Answer from the drawing. Dimensions are ordinates in mm from the lowest x, y and z of the part. Give positions to 0.01 mm unless a question says otherwise; leave off trailing zeros. Order: outer loops, then holes, each group sorted by start corner. A loop starts at its lowest first (then second) coordinate and runs counter-clockwise, first axis right, second up. Notation, with made-up numbers: (12.5, -6.5) - (22.5, -6.5) arc R17 ccw to (22.5, 23.5) - close; hole circle Ø2 at (-38, 72). An arc over 180 degrees is marked (long way). Use a Markdown table: item, result. Add a question column.
1) Find section D-D, the plane x = 190. Determine the outline of the cut face in (y, z), plus the area to 3 significant figures.
2) Find section C-C, the plane x = 99. Determine the outline of the cut face in (y, z).
3) Find section A-A, the plane y = 153. Determine the outline of the cut face in (x, z), plus the area to 3 significant figures.
4) Straight lines are drawn through the part: line 1 (X direction, y = 30.5, z = 18.25) (1 decimal); line 2 (Y direction, x = 70.5, z = 16) (1 decimal); line 3 (Y direction, x = 91, z = 14.75) (1 decimal). For each, find the intervals that lie inside material, in ascending order.
5) Flat-ended cylindrical pins translate along their axes: pin 1 (3 mm diameter, centred on x = 240, y = 183.5, fed in from +Z); pin 2 (5.5 mm diameter, centred on y = 139.5, z = 7.5, fed in from +X); pin 3 (2 mm diameter, centred on y = 118, z = 5, fed in from +X). Find the tip coordinate at first contact, or state that the pin passes through.
6) The mould has two halves that part along X. Classify the marked faces 1, 2 and 3: released by +X, released by -X, zero draft, split by the parting line, or undercut.
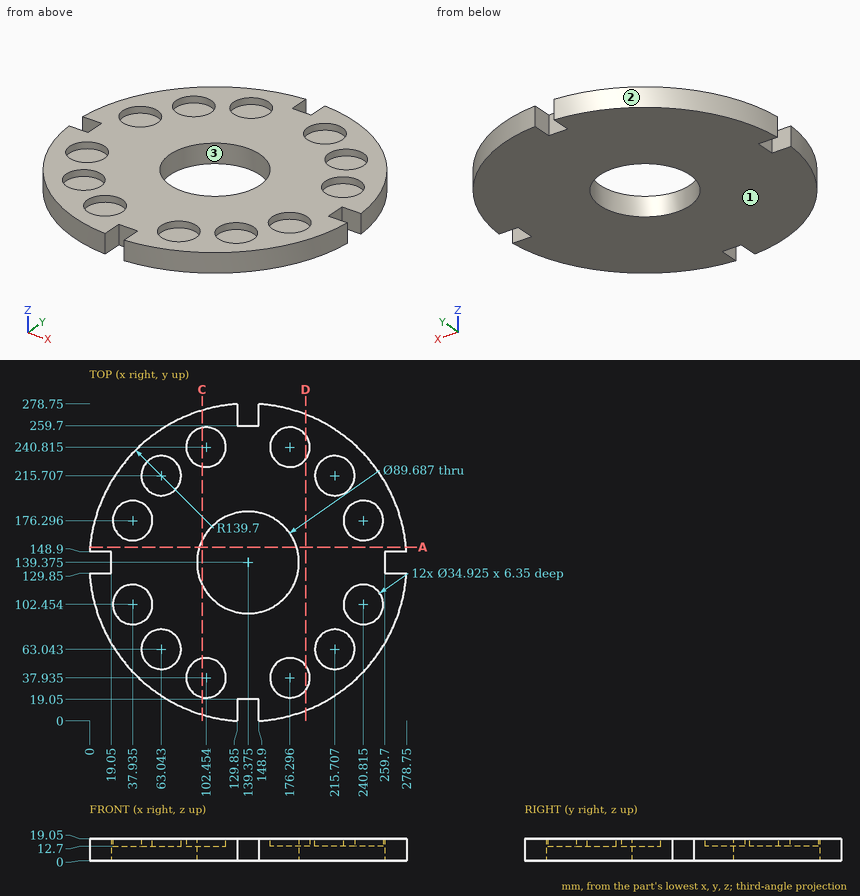
The answers:
| question | item | result |
|---|---|---|
| 1 | outline | (9.17, 0) - (269.58, 0) - (269.58, 19.05) - (251.64, 19.05) - (251.64, 12.7) - (229.99, 12.7) - (229.99, 19.05) - (48.76, 19.05) - (48.76, 12.7) - (27.11, 12.7) - (27.11, 19.05) - (9.17, 19.05) - close |
| 1 | area | 4,690 mm2 |
| 2 | outline | (5.64, 0) - (119.86, 0) - (119.86, 19.05) - (55.05, 19.05) - (55.05, 12.7) - (20.82, 12.7) - (20.82, 19.05) - (5.64, 19.05) - close; (158.89, 0) - (273.11, 0) - (273.11, 19.05) - (257.93, 19.05) - (257.93, 12.7) - (223.7, 12.7) - (223.7, 19.05) - (158.89, 19.05) - close |
| 3 | outline | (0.34, 0) - (96.65, 0) - (96.65, 19.05) - (0.34, 19.05) - close; (182.1, 0) - (278.41, 0) - (278.41, 19.05) - (182.1, 19.05) - close |
| 3 | area | 3,670 mm2 |
| 4 | line 1 | 51.8 to 86.7, 118.3 to 160.5, 192.1 to 226.9 |
| 4 | line 2 | 17.8 to 47.3, 78.8 to 199.9, 231.5 to 260.9 |
| 4 | line 3 | 8.3 to 24.8, 51.1 to 227.6, 254 to 270.4 |
| 5 | pin 1 | z = 12.7 |
| 5 | pin 2 | x = 259.7 |
| 5 | pin 3 | x = 277.58 |
| 6 | face 1 | zero draft |
| 6 | face 2 | released by -X |
| 6 | face 3 | undercut |
